Can you work these out from the model? Positions are in its coordinate system, mm. Face numbers are marked on the shaded views. Coordinates: 2 decimals unless noted, no trailing zeros. Write each loop counter-clockwise with the first axis right and the second up, starting at its lowest first coordinate (ties: lowest second). Pieces come first, ordered by that corner, then holes.
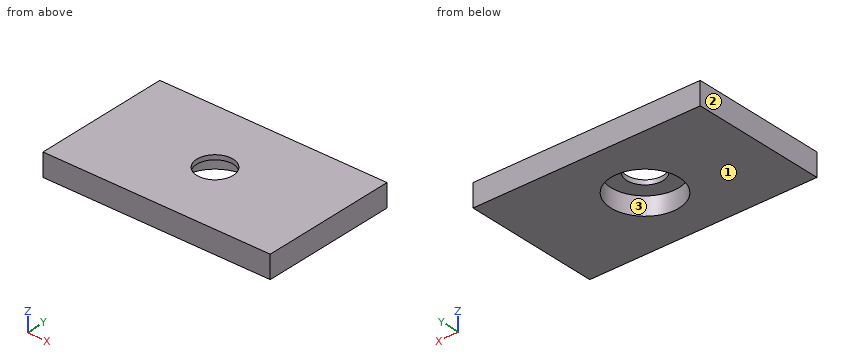
```python
from build123d import *

# Parameters (mm, degrees)
SKETCH_W     = 50
SKETCH_H     = 30
SKETCH_R     = 7.5
PAD_DEPTH    = 4
SKETCH001_W  = 50
SKETCH001_H  = 30
SKETCH001_R  = 4
PAD001_DEPTH = 1


with BuildPart() as part:
    # Sketch → Pad (new body)
    with BuildSketch(Plane.XY):
        with Locations((25, 15)):
            Rectangle(SKETCH_W, SKETCH_H)
        with Locations((25, 15)):
            Circle(SKETCH_R, mode=Mode.SUBTRACT)
    extrude(amount=PAD_DEPTH)

    # Sketch001 (on Face7 of Pad) → Pad001 (join)
    with BuildSketch(Plane.XY.offset(4)):
        with Locations((25, 15)):
            Rectangle(SKETCH001_W, SKETCH001_H)
        with Locations((25, 15)):
            Circle(SKETCH001_R, mode=Mode.SUBTRACT)
    extrude(amount=PAD001_DEPTH)


solid = part.part
```
1. If we section it at A-A, the plane y = 15: List the corners of the cut face in (x, z) for me.
2. If we section it at D-D, the plane y = 8.25: List the corners of the cut face in (x, z) for me.
3. If I drill on L1, parallel to Y at x = 25, z = 1.85; L2, parallel to Y at x = 25, z = 4.85; L3, parallel to X at y = 11.5, z = 1, over which ranges is the centre line in solid material (lowest first)?
4. If we section it at B-B, the plane x = 25: List the corners of the cut face in (y, z) for me, plus the area to 3 significant figures.
5. I'm going to push flat-ended pins straight in: P1, Ø12, axis at x = 25, y = 15, coming from the -Z side; P2, Ø2, axis at x = 33, y = 9.5, coming from the -Z side. Where does each tip first touch, or does it pass through?
6. If we section it at C-C, the plane z = 2.95: List the corners of the cut face in (x, y) for me, plus the area to 3 significant figures.
7. We'd pull the mould along X, two halves only. Please class the marked faces 1, 2 and 3: released by +X, released by -X, zero draft, split by the parting line, or undercut.
Answers:
1. outline: (0, 0) - (17.5, 0) - (17.5, 4) - (21, 4) - (21, 5) - (0, 5) - close; (29, 4) - (32.5, 4) - (32.5, 0) - (50, 0) - (50, 5) - (29, 5) - close
2. outline: (0, 0) - (21.73, 0) - (21.73, 4) - (28.27, 4) - (28.27, 0) - (50, 0) - (50, 5) - (0, 5) - close
3. L1: y = 0 to 7.5, 22.5 to 30
3. L2: y = 0 to 11, 19 to 30
3. L3: x = 0 to 18.37, 31.63 to 50
4. outline: (0, 0) - (7.5, 0) - (7.5, 4) - (11, 4) - (11, 5) - (0, 5) - close; (19, 4) - (22.5, 4) - (22.5, 0) - (30, 0) - (30, 5) - (19, 5) - close
4. area: 82.0 mm2
5. P1: stops at z = 4
5. P2: stops at z = 0
6. outline: (0, 0) - (50, 0) - (50, 30) - (0, 30) - close; hole circle Ø15 at (25, 15)
6. area: 1,320 mm2
7. face 1: zero draft
7. face 2: released by -X
7. face 3: undercut
